Could you check a few things on this model? Use its own coordinates, in mm. A direction names the side the tool comes from. Coordinates: 2 decimals unless noted, no trailing zeros. Order: outer loops, then holes, each group sorted by start corner. A loop starts at its lowest first (then second) coordinate and runs counter-clockwise, first axis right, second up. Notation, with made-up numbers: (19.25, 53) - (33.25, 53) arc R28 ccw to (33.25, 87) - close; hole circle Ø8 at (30, -28). An arc over 180 degrees is marked (long way). One line per item, written item: value.
from build123d import *

# Parameters (mm, degrees)
CROQUIS1_R              = 1.707370132
SALIENTE_EXTRUIR1_DEPTH = 9.5
SALIENTE_EXTRUIR2_DEPTH = 2.5
CROQUIS5_R              = 4
CROQUIS5_R_2            = 3.5
CORTAR_EXTRUIR1_DEPTH   = 2.5
REDONDEO1_R             = 3
CROQUIS6_R              = 3.1
CORTAR_EXTRUIR2_DEPTH   = 7.5


with BuildPart() as part:
    # Croquis1 → Saliente-Extruir1 (new body)
    with BuildSketch(Plane.XY):
        Polygon((-69.586479396, 30.699597615), (-44.586479396, 30.699597615), (-44.586479396, -7.300402385), (-69.586479396, -7.300402385), (-74.586479396, -4.300402385), (-74.586479396, 27.699597615), align=None)
        with Locations((-69.586479396, 27.699597615)):
            Circle(CROQUIS1_R, mode=Mode.SUBTRACT)
        with Locations((-69.586479396, -4.300402385)):
            Circle(CROQUIS1_R, mode=Mode.SUBTRACT)
    extrude(amount=SALIENTE_EXTRUIR1_DEPTH)

    # Croquis4 → Saliente-Extruir2 (add)
    with BuildSketch(Plane.XY.offset(9.5)):
        Polygon((-72.086479396, 29.199597615), (-117.086479396, 29.199597615), (-117.086479396, -5.800402385), (-72.086479396, -5.800402385), (-74.586479396, -4.300402385), (-74.586479396, 27.699597615), align=None)
    extrude(amount=-SALIENTE_EXTRUIR2_DEPTH)

    # Croquis5 → Cortar-Extruir1 (cut)
    with BuildSketch(Plane.XY.offset(9.5)):
        with Locations((-91.086479396, -4.300402385)):
            Circle(CROQUIS5_R)
        with Locations((-91.086479396, 27.699597615)):
            Circle(CROQUIS5_R)
        with Locations((-121.586479396, -4.300402385)):
            Circle(CROQUIS5_R_2)
        with Locations((-121.586479396, 27.699597615)):
            Circle(CROQUIS5_R_2)
        with Locations((-100.336479396, 19.699597615)):
            Circle(CROQUIS5_R)
        with Locations((-112.336479396, 19.699597615)):
            Circle(CROQUIS5_R)
        with Locations((-112.336479396, 3.699597615)):
            Circle(CROQUIS5_R)
        with Locations((-100.336479396, 3.699597615)):
            Circle(CROQUIS5_R)
    extrude(amount=-CORTAR_EXTRUIR1_DEPTH, mode=Mode.SUBTRACT)

    # Redondeo1
    redondeo1_edges = [part.edges().sort_by_distance(p)[0] for p in [
        (-44.586479396, 30.699597615, 4.75),
        (-44.586479396, -7.300402385, 4.75),
        (-117.086479396, -5.800402385, 8.25),
        (-117.086479396, 29.199597615, 8.25),
    ]]
    fillet(redondeo1_edges, radius=REDONDEO1_R)

    # Croquis6 → Cortar-Extruir2 (cut)
    with BuildSketch(Plane.XY.offset(9.5)):
        with Locations((-69.586479396, 27.699597615)):
            Circle(CROQUIS6_R)
        with Locations((-69.586479396, -4.300402385)):
            Circle(CROQUIS6_R)
    extrude(amount=-CORTAR_EXTRUIR2_DEPTH, mode=Mode.SUBTRACT)


solid = part.part
Item 1: If I drill on probe 1 along X at (y, z) = (18, 8.5); probe 2 along X at (y, z) = (23, 8); probe 3 along X at (y, z) = (1, 4.5), over which ranges is the centre line in solid material (lowest first)?
Conclusion:
probe 1: -117.09 to -115.96, -108.72 to -103.96, -96.72 to -44.59
probe 2: -117.09 to -114.6, -110.08 to -102.6, -98.08 to -44.59
probe 3: -74.59 to -44.59
Item 2: I'm going to push flat-ended pins straight in: pin 1 Ø3.5 at (x, y) = (-69.59, 27.7) entering from +Z; pin 2 Ø1.2 at (x, z) = (-105.5, 8) entering from +Y; pin 3 Ø1 at (y, z) = (-3, 4.5) entering from -X. Where does each tip first touch, or does it pass through?
Conclusion:
pin 1: z = 2
pin 2: y = 29.2
pin 3: x = -74.59
Item 3: For faces 1 (the face through (-72.677, 28.845, 2.673)), 2 (the face through (-105, -5.8, 8)), 3 (the face through (-80, 29.2, 8)), 4 (the face through (-68.46, 24.81, 5.8)), 5 (the face through (-116.333, 3.875, 8.268)), which set-ups out of +Z, -Z, +X, -X, +Y, -Y let a thin tool reach every point of the face, with its end or its side?
Conclusion:
face 1: -Z, -X, +Y
face 2: +Z, -Z, -X, -Y
face 3: +Z, -Z, -X, +Y
face 4: +Z
face 5: +Z, -Z
Item 4: I want a section at A-A on z = 1. Please give me the cut outline in (x, y), then the cut area to 3 significant figures.
Conclusion:
outline: (-74.59, -4.3) - (-69.59, -7.3) - (-47.59, -7.3) arc R3 ccw to (-44.59, -4.3) - (-44.59, 27.7) arc R3 ccw to (-47.59, 30.7) - (-69.59, 30.7) - (-74.59, 27.7) - close; hole circle Ø3.41 at (-69.59, -4.3); hole circle Ø3.41 at (-69.59, 27.7)
area: 1,100 mm²
Item 5: Thinking about a two-plate mould opening in Y: for faces 6 (the face through (-68.265, -1.496, 5.802)), 7 (the face through (-96.64, 2.17, 8.27)), 8 (the face through (-104, 29.2, 8)), 9 (the face through (-44.586, 12, 5)), which applies, pulls with the +Y half, pulls with the -Y half, needs draft (parallel to the pull), parting line crosses it, or undercut?
Conclusion:
face 6: undercut
face 7: undercut
face 8: pulls with the +Y half
face 9: needs draft
Item 6: I want a section at B-B on x = -112. Please give me the cut outline in (y, z).
Conclusion:
outline: (-5.8, 7) - (-0.29, 7) - (-0.29, 9.5) - (-5.8, 9.5) - close; (7.69, 7) - (15.71, 7) - (15.71, 9.5) - (7.69, 9.5) - close; (23.69, 7) - (29.2, 7) - (29.2, 9.5) - (23.69, 9.5) - close
Item 7: I want a section at D-D on y = 14. Please give me the cut outline in (x, z).
Conclusion:
outline: (-117.09, 7) - (-74.59, 7) - (-74.59, 0) - (-44.59, 0) - (-44.59, 9.5) - (-117.09, 9.5) - close
Item 8: I want a section at C-C on y = 20.5. Please give me the cut outline in (x, z), then the cut area to 3 significant figures.
Conclusion:
outline: (-117.09, 7) - (-116.26, 7) - (-116.26, 9.5) - (-117.09, 9.5) - close; (-108.42, 7) - (-104.26, 7) - (-104.26, 9.5) - (-108.42, 9.5) - close; (-96.42, 7) - (-74.59, 7) - (-74.59, 0) - (-44.59, 0) - (-44.59, 9.5) - (-96.42, 9.5) - close
area: 352 mm²
